Model file for the job. Use its own axes, mm. A direction names the side the tool comes from. Give positions to 0.01 mm unless a question says otherwise; leave off trailing zeros. Write each loop counter-clockwise with the first axis right and the second up, starting at its lowest first coordinate (ties: lowest second). Pieces come first, ordered by that corner, then holes. Notation, with made-up numbers: (35, -33.5) - (68, -33.5) arc R37 cw to (68, 4.5) - close; hole circle Ø6 at (26.5, 54.5). An arc over 180 degrees is marked (long way). Use a Markdown table: item, result. Add a question column.
```python
from build123d import *
from build123d.topology import SkipClean

# Parameters (mm, degrees)
SKETCH2_W               = 14
SKETCH2_H               = 6
BOSS_EXTRUDE1_DEPTH     = 4
SKETCH3_W               = 4
SKETCH3_H               = 6
BOSS_EXTRUDE2_DEPTH     = 12
CUT_EXTRUDE1_DEPTH      = 22.470910554
CUT_EXTRUDE1_DEPTH_BACK = 22.470910554
SKETCH4_R               = 1.5
BOSS_EXTRUDE3_START     = 1
SKETCH5_R               = 2.5
SKETCH5_R_2             = 1.5
BOSS_EXTRUDE3_DEPTH     = 1
SKETCH6_R               = 2.5
SKETCH6_R_2             = 1.5
BOSS_EXTRUDE4_DEPTH     = 1
SKETCH7_W               = 4
SKETCH7_H               = 6
SKETCH7_R               = 1
BOSS_EXTRUDE5_DEPTH     = 4
FILLET1_R               = 2
FILLET2_R               = 3


with BuildPart() as part:
    # Sketch2 → Boss-Extrude1 (new body)
    with BuildSketch(Plane(origin=(0, 0, 0), x_dir=(1, 0, 0), z_dir=(0, 1, 0))):
        Rectangle(SKETCH2_W, SKETCH2_H)
    extrude(amount=BOSS_EXTRUDE1_DEPTH)

    # Sketch3 → Boss-Extrude2 (add)
    with BuildSketch(Plane(origin=(0, 4, 0), x_dir=(1, 0, 0), z_dir=(0, 1, 0))):
        with Locations((-5, 0)):
            Rectangle(SKETCH3_W, SKETCH3_H)
        with Locations((5, 0)):
            Rectangle(SKETCH3_W, SKETCH3_H)
    extrude(amount=BOSS_EXTRUDE2_DEPTH)

    # Sketch4 → Cut-Extrude1 (cut, two sides: drawn at the far end of the back side and taken through both)
    with BuildSketch(Plane(origin=(7, 0, 0), x_dir=(0, 0, -1), z_dir=(1, 0, 0)).offset(-CUT_EXTRUDE1_DEPTH_BACK)):
        with Locations((0, 12)):
            Circle(SKETCH4_R)
    extrude(amount=CUT_EXTRUDE1_DEPTH + CUT_EXTRUDE1_DEPTH_BACK, mode=Mode.SUBTRACT)

    # Sketch5 → Boss-Extrude3 (add)
    with BuildSketch(Plane(origin=(-3, 0, 0), x_dir=(0, 0, -1), z_dir=(1, 0, 0)).offset(BOSS_EXTRUDE3_START)):
        with Locations(Location((0, 12, 0), (0, 0, 180))):
            Circle(SKETCH5_R)
        with Locations((0, 12)):
            Circle(SKETCH5_R_2, mode=Mode.SUBTRACT)
    extrude(amount=-BOSS_EXTRUDE3_DEPTH)

    # Sketch6 → Boss-Extrude4 (add)
    with SkipClean():  # the faces are left unmerged after this step: merging them gives an invalid solid
        with BuildSketch(Plane.ZY.offset(-3)):
            with Locations((0, 12)):
                Circle(SKETCH6_R)
            with Locations((0, 12)):
                Circle(SKETCH6_R_2, mode=Mode.SUBTRACT)
        extrude(amount=BOSS_EXTRUDE4_DEPTH)

    # Sketch7 → Boss-Extrude5 (add)
    # profile 1 of 2: a face of its own
    with SkipClean():  # the faces are left unmerged after this step: merging them gives an invalid solid
        with BuildSketch(Plane(origin=(0, 4, 0), x_dir=(1, 0, 0), z_dir=(0, 1, 0))):
            with Locations((9, 0)):
                Rectangle(SKETCH7_W, SKETCH7_H)
            with Locations(Location((9, 0, 0), (0, 0, 270))):
                Circle(SKETCH7_R, mode=Mode.SUBTRACT)
        # profile 2 of 2: a face of its own
        with BuildSketch(Plane(origin=(0, 4, 0), x_dir=(1, 0, 0), z_dir=(0, 1, 0))):
            with Locations((-9, 0)):
                Rectangle(SKETCH7_W, SKETCH7_H)
            with Locations(Location((-9, 0, 0), (0, 0, 270))):
                Circle(SKETCH7_R, mode=Mode.SUBTRACT)
        extrude(amount=-BOSS_EXTRUDE5_DEPTH)

    # Fillet1
    fillet1_edges = [part.edges().sort_by_distance(p)[0] for p in [
        (11, 2, -3),
        (11, 2, 3),
        (-11, 2, 3),
        (-11, 2, -3),
    ]]
    fillet(fillet1_edges, radius=FILLET1_R)

    # Fillet2
    fillet2_edges = [part.edges().sort_by_distance(p)[0] for p in [
        (-5, 16, -3),
        (5, 16, -3),
        (5, 16, 3),
        (-5, 16, 3),
    ]]
    fillet(fillet2_edges, radius=FILLET2_R - 0.0001)  # a hair under: the kernel refuses the full size


solid = part.part
```
(1) Band-saw the part on B-B (x = -2.75). Write the cut outline in (y, z), then the cut area to 3 significant figures.
(2) Band-saw the part on A-A (y = 12). Write the cut outline in (x, z).
(3) Which spindle directions (+Z, -Z, +X, -X, +Y, -Y) get a long thin tool onto all of the face, cutting with end or side? Do faces 5 (the cylindrical face through (5.03, 15.1, 2.14)), 6 (the cylindrical face through (10, 2, 0)), 7 (the cylindrical face through (2.51, 9.56, -0.54)), 8 (the flat face through (2, 10, 0)), 9 (the flat face through (7, 10, 0)). Say none if no direction does.
(4) Flat gauge pins, fed straight in: pin 1 (2.5 mm diameter, centred on y = 12, z = 0, fed in from -X); pin 2 (3 mm diameter, centred on x = -9, z = 1, fed in from +Y); pin 3 (3 mm diameter, centred on y = 7.5, z = 1.5, fed in from -X). Where does each tip first touch, or does it go through?
(5) Two-plate mould, pull along X, no slides. Class faces 1 (the flat face through (-3, 9, 0)), 2 (the cylindrical face through (-10.43, 1.97, -2.4)), 3 (the flat face through (8, 4, 1)), 4 (the cylindrical face through (-8, 2, 0)): +X half, -X half, draft (parallel to the pull), parting line (faces both ways), or undercut.
(6) Probe probe 1 along Y at (x, z) = (-2.5, 0); probe 2 along X at (y, z) = (1.5, 0); probe 3 along Y at (x, z) = (2.5, 0.5). List the from-to ranges inside material, lowest first. Write a range as [from, to].
(7) Band-saw the part on C-C (z = 1.25). Write the cut outline in (x, y).
(8) Band-saw the part on D-D (y = 1). Write the cut outline in (x, z).
Model answer:
| question | item | result |
|---|---|---|
| 1 | outline | (0, -3) - (4, -3) - (4, 3) - (0, 3) - close; circle Ø5 at (12, 0); hole circle Ø3 at (12, 0) |
| 1 | area | 36.6 mm^2 |
| 2 | outline | (-7, -3) - (-3, -3) - (-3, -2.5) - (-2, -2.5) - (-2, -1.5) - (-7, -1.5) - close; (-7, 1.5) - (-2, 1.5) - (-2, 2.5) - (-3, 2.5) - (-3, 3) - (-7, 3) - close; (2, -2.5) - (3, -2.5) - (3, -3) - (7, -3) - (7, -1.5) - (2, -1.5) - close; (2, 1.5) - (7, 1.5) - (7, 3) - (3, 3) - (3, 2.5) - (2, 2.5) - close |
| 3 | face 5 | +Z, +X, -X, +Y |
| 3 | face 6 | +Y, -Y |
| 3 | face 7 | none |
| 3 | face 8 | +Z, -Z, +Y |
| 3 | face 9 | +Z, -Z, +X, +Y |
| 4 | pin 1 | passes through |
| 4 | pin 2 | stops at y = 4 |
| 4 | pin 3 | stops at x = -7 |
| 5 | face 1 | undercut |
| 5 | face 2 | -X half |
| 5 | face 3 | draft |
| 5 | face 4 | undercut |
| 6 | probe 1 | y = [0, 4], [9.5, 10.5], [13.5, 14.5] |
| 6 | probe 2 | x = [-11, -10], [-8, 8], [10, 11] |
| 6 | probe 3 | y = [0, 4], [9.55, 10.59], [13.41, 14.45] |
| 7 | outline | (-10.98, 0) - (10.98, 0) - (10.98, 4) - (7, 4) - (7, 11.17) - (2, 11.17) - (2, 9.83) - (3, 9.83) - (3, 4) - (-3, 4) - (-3, 9.83) - (-2, 9.83) - (-2, 11.17) - (-7, 11.17) - (-7, 4) - (-10.98, 4) - close; (-7, 12.83) - (-2, 12.83) - (-2, 14.17) - (-3, 14.17) - (-3, 15.73) - (-7, 15.73) - close; (2, 12.83) - (7, 12.83) - (7, 15.73) - (3, 15.73) - (3, 14.17) - (2, 14.17) - close |
| 8 | outline | (-11, -1) arc R2 ccw to (-9, -3) - (9, -3) arc R2 ccw to (11, -1) - (11, 1) arc R2 ccw to (9, 3) - (-9, 3) arc R2 ccw to (-11, 1) - close; hole circle Ø2 at (-9, 0); hole circle Ø2 at (9, 0) |
